```python
from build123d import *

# Parameters (mm, degrees)
CUT_EXTRUDE_1_DEPTH = 2


with BuildPart() as part:
    # ｽｹｯﾁ2 → 回転1 (revolve)
    with BuildSketch(Plane.XY, mode=Mode.PRIVATE) as revolve_1_sk:
        Polygon((0, 6), (0, 0), (96.2, 0), (96.2, 6), (95.2, 6), (95.2, 5.5), (94.2, 5.5), (94.2, 6), (2, 6), (1, 6), align=None)
    revolve(revolve_1_sk.sketch.rotate(Axis((0, 0, 0), (1, 0, 0)), 90), axis=Axis((0, 0, 0), (1, 0, 0)))

    # ｽｹｯﾁ4 → ｶｯﾄ - 押し出し1 (cut)
    with BuildSketch(Plane(origin=(0, 6, 0), x_dir=(1, 0, 0), z_dir=(0, 1, 0))):
        with BuildLine():
            Line((5, 2), (10, 2))
            ThreePointArc((10, 2), (12, 0), (10, -2))
            Line((10, -2), (5, -2))
            ThreePointArc((5, -2), (3, 0), (5, 2))
        make_face()
        with BuildLine():
            Line((75, -2), (70, -2))
            ThreePointArc((70, -2), (68, 0), (70, 2))
            Line((70, 2), (75, 2))
            ThreePointArc((75, 2), (77, 0), (75, -2))
        make_face()
    extrude(amount=-CUT_EXTRUDE_1_DEPTH, mode=Mode.SUBTRACT)


solid = part.part
```
Geometry: final body of the model. Coordinates: model frame, mm. A direction names the side the tool comes from. Coordinates: 2 decimals unless noted, no trailing zeros. Loops run counter-clockwise (first coordinate to the right, second up) from the corner with the lowest first, then second, coordinate; pieces in that order, holes last. Notation, with made-up numbers: (3, -35) -> (18, -35) arc R28 ccw to (18, -11) -> close; hole circle Ø2 at (55, -1.75). An arc over 180 degrees is marked (long way). Use a Markdown table: item, result. Add a question column.
(1) Line query: line 1 along X through (y, z) = (4.75, 1.5); line 2 along Z through (x, y) = (77, -0.5); line 3 along Y through (x, z) = (64, 0.75). Output: solid intervals per line, ascending.
(2) Access query for faces 4 (the flat face through (73, 4, 0)), 5 (the flat face through (95.2, 5, 3)), 6 (the cylindrical face through (46.441, -5.059, 3.226)). Directions: +Z, -Z, +X, -X, +Y, -Y. A direction counts if a zero-diameter tool reaches every point of the face in a straight line with its end or side. Return the directions, or none.
(3) Section query C-C, the plane x = 25.5. Return loops of the section in (y, z).
(4) Mould query, pull axis X, two halves, no side actions, for faces 1 (the cylindrical face through (95.693, -1.802, 5.723)), 2 (the flat face through (73, 5, 2)), 3 (the flat face through (96.2, 0, 0)). Classes: pulls with the +X half, pulls with the -X half, needs draft (parallel to the pull), parting line crosses it, or undercut.
(5) Section query B-B, the plane y = 1.25. Return loops of the section in (x, z).
(6) Pin query (flat end, axial travel): pin 1 Ø2 at (x, z) = (73, -0.5) entering from +Y; pin 2 Ø0.5 at (x, y) = (8.5, 5) entering from +Z; pin 3 Ø1 at (x, y) = (23, -3.5) entering from +Z. Return the tip coordinate at first contact, or that it passes through.
(7) Section query A-A, the plane z = 0. Return loops of the section in (x, y), plus the area to 3 significant figures.
(8) Section query D-D, the plane z = 3.75. Return loops of the section in (x, y), plus the area to 3 significant figures.
Answer:
| question | item | result |
|---|---|---|
| 1 | line 1 | x = 0 to 3.68, 11.32 to 68.68, 76.32 to 96.2 |
| 1 | line 2 | z = -5.98 to 5.98 |
| 1 | line 3 | y = -5.95 to 5.95 |
| 2 | face 4 | +Y |
| 2 | face 5 | none |
| 2 | face 6 | +X, -X |
| 3 | outline | circle Ø12 at (0, 0) |
| 4 | face 1 | needs draft |
| 4 | face 2 | undercut |
| 4 | face 3 | pulls with the +X half |
| 5 | outline | (0, -5.87) -> (94.2, -5.87) -> (94.2, -5.36) -> (95.2, -5.36) -> (95.2, -5.87) -> (96.2, -5.87) -> (96.2, 5.87) -> (95.2, 5.87) -> (95.2, 5.36) -> (94.2, 5.36) -> (94.2, 5.87) -> (0, 5.87) -> close |
| 6 | pin 1 | stops at y = 4 |
| 6 | pin 2 | stops at z = 3.67 |
| 6 | pin 3 | stops at z = 5.2 |
| 7 | outline | (0, -6) -> (94.2, -6) -> (94.2, -5.5) -> (95.2, -5.5) -> (95.2, -6) -> (96.2, -6) -> (96.2, 6) -> (95.2, 6) -> (95.2, 5.5) -> (94.2, 5.5) -> (94.2, 6) -> (77, 6) -> (77, 4) -> (68, 4) -> (68, 6) -> (12, 6) -> (12, 4) -> (3, 4) -> (3, 6) -> (0, 6) -> close |
| 7 | area | 1,120 mm^2 |
| 8 | outline | (0, -4.68) -> (94.2, -4.68) -> (94.2, -4.02) -> (95.2, -4.02) -> (95.2, -4.68) -> (96.2, -4.68) -> (96.2, 4.68) -> (95.2, 4.68) -> (95.2, 4.02) -> (94.2, 4.02) -> (94.2, 4.68) -> (0, 4.68) -> close |
| 8 | area | 900 mm^2 |
